For this review, take the finished solid that the model builds, in its own axes (mm). Face numbers are marked on the shaded views. Coordinates: 2 decimals unless noted, no trailing zeros. Loops run counter-clockwise (first coordinate to the right, second up) from the corner with the lowest first, then second, coordinate; pieces in that order, holes last. Notation, with made-up numbers: (9.25, 81.25) -> (22.25, 81.25) arc R14 cw to (22.25, 88.25) -> close; hole circle Ø6 at (76, 62.5). An arc over 180 degrees is marked (long way). Use a Markdown table: item, result.
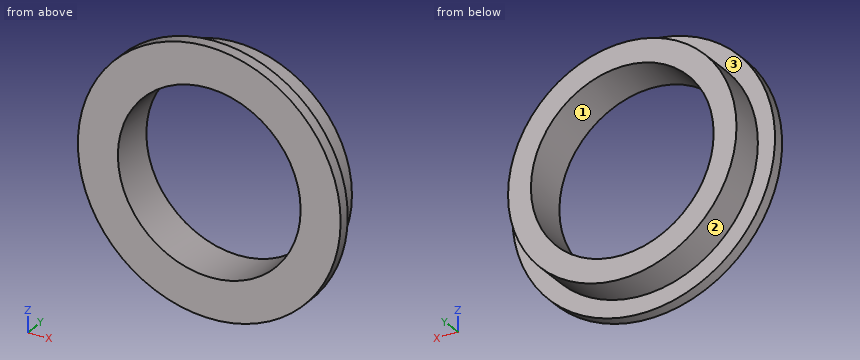
from build123d import *

# Parameters (mm, degrees)
SKETCH2_R           = 15.875
SKETCH2_R_2         = 12.7
BOSS_EXTRUDE1_DEPTH = 25.4
SKETCH3_R           = 18.25625
SKETCH3_R_2         = 15.875
BOSS_EXTRUDE2_DEPTH = 1.5875
SKETCH5_R           = 18.25625
CUT_EXTRUDE1_DEPTH  = 19.05


with BuildPart() as part:
    # Sketch2 → Boss-Extrude1 (new body)
    with BuildSketch(Plane(origin=(0, 0, 0), x_dir=(1, 0, 0), z_dir=(0, 1, 0))):
        Circle(SKETCH2_R)
        Circle(SKETCH2_R_2, mode=Mode.SUBTRACT)
    extrude(amount=BOSS_EXTRUDE1_DEPTH)

    # Sketch3 → Boss-Extrude2 (add)
    with BuildSketch(Plane(origin=(0, 0, 0), x_dir=(1, 0, 0), z_dir=(0, 1, 0))):
        Circle(SKETCH3_R)
        Circle(SKETCH3_R_2, mode=Mode.SUBTRACT)
    extrude(amount=BOSS_EXTRUDE2_DEPTH)

    # Sketch5 → Cut-Extrude1 (cut)
    with BuildSketch(Plane(origin=(0, 25.4, 0), x_dir=(1, 0, 0), z_dir=(0, 1, 0))):
        Circle(SKETCH5_R)
    extrude(amount=-CUT_EXTRUDE1_DEPTH, mode=Mode.SUBTRACT)


solid = part.part
(1) For line 1 along Z through (x, y) = (0, 3.75) (3 decimals); line 2 along Z through (x, y) = (0, 1.5), list the stretches that pass through material, from the lowest coordinate up.
Found:
| item | result |
|---|---|
| line 1 | z = -15.875 to -12.7, 12.7 to 15.875 |
| line 2 | z = -18.26 to -12.7, 12.7 to 18.26 |
(2) Take a section at C-C on y = 3. Write out the cut boundary in (x, z) (3 decimals).
Found:
| item | result |
|---|---|
| outline | circle Ø31.75 at (0, 0); hole circle Ø25.4 at (0, 0) |
(3) For pin 1 Ø1.5 at (x, y) = (-4.5, 3) entering from -Z; pin 2 Ø1.5 at (y, z) = (5.5, 13) entering from +X; pin 3 Ø3 at (x, y) = (4, 3) entering from -Z, all flat-tipped, find the tip position at first contact; note any pin that passes through.
Found:
| item | result |
|---|---|
| pin 1 | stops at z = -15.43 |
| pin 2 | stops at x = 10.1 |
| pin 3 | stops at z = -17.92 |
(4) Mouldability with a two-part tool opening along Z and no side actions: class the marked faces 1, 2 and 3 as pulls with the +Z half, pulls with the -Z half, needs draft (parallel to the pull), parting line crosses it, or undercut.
Found:
| item | result |
|---|---|
| face 1 | undercut |
| face 2 | parting line crosses it |
| face 3 | needs draft |
